from build123d import *

# Parameters (mm, degrees)
SKETCH1_R           = 25
BOSS_EXTRUDE1_DEPTH = 25
SKETCH2_R           = 9.5
CUT_EXTRUDE1_DEPTH  = 20
SKETCH3_R           = 6
CUT_EXTRUDE2_DEPTH  = 20
SKETCH4_W           = 31.902567833
SKETCH4_H           = 50
CUT_EXTRUDE3_DEPTH  = 26
SKETCH5_R           = 2.75
CUT_EXTRUDE4_DEPTH  = 26
CUT_EXTRUDE5_START  = -15
SKETCH6_R           = 5
CUT_EXTRUDE5_DEPTH  = 20
SKETCH7_R           = 1.75
CUT_EXTRUDE6_DEPTH  = 26.0000001
SKETCH8_R           = 3.5
CUT_EXTRUDE7_DEPTH  = 5


with BuildPart() as part:
    # Sketch1 → Boss-Extrude1 (new body)
    with BuildSketch(Plane.XY):
        Circle(SKETCH1_R)
    extrude(amount=BOSS_EXTRUDE1_DEPTH)

    # Sketch2 → Cut-Extrude1 (cut)
    with BuildSketch(Plane.XY.offset(25)):
        Circle(SKETCH2_R)
    extrude(amount=-CUT_EXTRUDE1_DEPTH, mode=Mode.SUBTRACT)

    # Sketch3 → Cut-Extrude2 (cut)
    with BuildSketch(Plane.XY.offset(5)):
        Circle(SKETCH3_R)
    extrude(amount=-CUT_EXTRUDE2_DEPTH, mode=Mode.SUBTRACT)

    # Sketch4 → Cut-Extrude3 (cut, through all)
    with BuildSketch(Plane.XY.offset(25)):
        with Locations((-15.951283917, 0)):
            Rectangle(SKETCH4_W, SKETCH4_H)
    extrude(amount=-CUT_EXTRUDE3_DEPTH, mode=Mode.SUBTRACT)

    # Sketch5 → Cut-Extrude4 (cut, through all)
    with BuildSketch(Plane.ZY):
        with Locations((12.5, -14.5)):
            Circle(SKETCH5_R)
        with Locations((12.5, 14.5)):
            Circle(SKETCH5_R)
    extrude(amount=-CUT_EXTRUDE4_DEPTH, mode=Mode.SUBTRACT)

    # Sketch6 → Cut-Extrude5 (cut)
    with BuildSketch(Plane.ZY.offset(CUT_EXTRUDE5_START)):
        with Locations((12.5, 14.5)):
            Circle(SKETCH6_R)
        with Locations((12.5, -14.5)):
            Circle(SKETCH6_R)
    extrude(amount=-CUT_EXTRUDE5_DEPTH, mode=Mode.SUBTRACT)

    # Sketch7 → Cut-Extrude6 (cut, through all)
    with BuildSketch(Plane.XY.offset(25)):
        with Locations((0, 21)):
            Circle(SKETCH7_R)
        with Locations((0, -21)):
            Circle(SKETCH7_R)
    extrude(amount=-CUT_EXTRUDE6_DEPTH, mode=Mode.SUBTRACT)

    # Sketch8 → Cut-Extrude7 (cut)
    with BuildSketch(Plane(origin=(0, 0, 0), x_dir=(-1, 0, 0), z_dir=(0, 0, -1))):
        with Locations((0, 21)):
            Circle(SKETCH8_R)
        with Locations((0, -21)):
            Circle(SKETCH8_R)
    extrude(amount=-CUT_EXTRUDE7_DEPTH, mode=Mode.SUBTRACT)


solid = part.part
CAD build for the part. Positions are in the model's coordinates, mm. A direction names the side the tool comes from. Coordinates: 2 decimals unless noted, no trailing zeros. Write each loop counter-clockwise with the first axis right and the second up, starting at its lowest first coordinate (ties: lowest second). Pieces come first, ordered by that corner, then holes. Notation, with made-up numbers: (-15.5, 74.5) - (20.5, 74.5) arc R24 ccw to (20.5, 102.5) - close; hole circle Ø5 at (66, 86.5). An arc over 180 degrees is marked (long way). Use a Markdown table: item, result. Add a question column.
Item 1: 3-axis set-ups, long thin cutter, end or side, ignore diameter. For faces 1 (the face through (2, 21, 5)), 2 (the face through (1.75, 20.96, 15.14)), 3 (the face through (7, 0, 5)), 4 (the face through (18.1, 9.62, 11.42)): which of +Z, -Z, +X, -X, +Y, -Y reach the whole face in a straight line?
Item 2: Drill centre lines: L1, parallel to Z at x = 18.75, y = -14.5; L2, parallel to Y at x = 7.75, z = 12.5; L3, parallel to Y at x = 12, z = 12.5. Where is each one in solid material? Low to high. Write a range as from..to.
Item 3: Band-saw the part on B-B, the plane y = 15.5. Give the cut face in (x, z).
Item 4: Band-saw the part on C-C, the plane x = 10.5. Give the cut face in (y, z), and give its area (3 significant figures).
Item 5: Band-saw the part on A-A, the plane z = 4. Give the cut face in (x, y).
Item 6: Mould opens along Y. For faces 5 (the face through (24.994, -0.55, 12.325)), 6 (the face through (6, 0, 3)), 7 (the face through (0, 24, 15)) say: pulls with the +Y half, pulls with the -Y half, needs draft (parallel to the pull), parting line crosses it, or undercut.
Item 7: Flat gauge pins, fed straight in: pin 1 (1 mm diameter, centred on x = 19, z = 4.5, fed in from +Y); pin 2 (4 mm diameter, centred on x = 9.5, z = 18.5, fed in from -Y); pin 3 (5 mm diameter, centred on x = 8, z = 19, fed in from +Y); pin 4 (4.5 mm diameter, centred on y = 14.5, z = 12.5, fed in from +X). Where does each tip first touch, or does it go through?
Item 8: Band-saw the part on D-D, the plane z = 12.5. Give the cut face in (x, y).
Numbers:
| question | item | result |
|---|---|---|
| 1 | face 1 | -Z, -X |
| 1 | face 2 | +Z, -Z, -X |
| 1 | face 3 | +Z, -X |
| 1 | face 4 | +X |
| 2 | L1 | 0..7.5, 17.5..25 |
| 2 | L2 | -23.77..-17.25, -11.75..-5.49, 5.49..11.75, 17.25..23.77 |
| 2 | L3 | -21.93..-17.25, -11.75..11.75, 17.25..21.93 |
| 3 | outline | (0, 0) - (19.62, 0) - (19.62, 7.6) - (15, 7.6) - (15, 9.94) - (0, 9.94) - close; (0, 15.06) - (15, 15.06) - (15, 17.4) - (19.62, 17.4) - (19.62, 25) - (0, 25) - close |
| 4 | outline | (-22.69, 0) - (22.69, 0) - (22.69, 25) - (-22.69, 25) - close; hole circle Ø5.5 at (-14.5, 12.5); hole circle Ø5.5 at (14.5, 12.5) |
| 4 | area | 1,090 mm2 |
| 5 | outline | (0, -25) arc R25 ccw to (0, 25) - (0, 24.5) arc R3.5 cw to (0, 17.5) - (0, 6) arc R6 cw to (0, -6) - (0, -17.5) arc R3.5 cw to (0, -24.5) - close |
| 6 | face 5 | parting line crosses it |
| 6 | face 6 | undercut |
| 6 | face 7 | needs draft |
| 7 | pin 1 | y = 16.82 |
| 7 | pin 2 | y = -23.85 |
| 7 | pin 3 | y = 24.39 |
| 7 | pin 4 | through |
| 8 | outline | (0, -25) arc R25 ccw to (15.64, -19.5) - (15, -19.5) - (15, -17.25) - (0, -17.25) - (0, -19.25) arc R1.75 cw to (0, -22.75) - close; (0, -11.75) - (15, -11.75) - (15, -9.5) - (23.12, -9.5) arc R25 ccw to (23.12, 9.5) - (15, 9.5) - (15, 11.75) - (0, 11.75) - (0, 9.5) arc R9.5 cw to (0, -9.5) - close; (0, 17.25) - (15, 17.25) - (15, 19.5) - (15.64, 19.5) arc R25 ccw to (0, 25) - (0, 22.75) arc R1.75 cw to (0, 19.25) - close |
